Geometry: final body of the model. Coordinates: model frame, mm. Coordinates: 2 decimals unless noted, no trailing zeros. Loops run counter-clockwise (first coordinate to the right, second up) from the corner with the lowest first, then second, coordinate; pieces in that order, holes last. Notation, with made-up numbers: (76.5, 28) - (102.5, 28) arc R27 ccw to (102.5, 46) - close; hole circle Ø1 at (-28, 86.5). An arc over 180 degrees is marked (long way). Answer in a Markdown table with one row per item.
from build123d import *

# Parameters (mm, degrees)
SKETCH_1_W      = 3
SKETCH_1_H      = 30
EXTRUDE_1_DEPTH = 0.6


with BuildPart() as part:
    # Эскиз1 → Бобышка-Вытянуть1 (new body)
    with BuildSketch(Plane(origin=(0, 0, 0), x_dir=(1, 0, 0), z_dir=(0, 1, 0))):
        Polygon((0, 78), (0, 0), (98, 0), (98, 78), (50.5, 78), (50.5, 48), (47.5, 48), (47.5, 78), align=None)
        with Locations((49, 93)):
            Rectangle(SKETCH_1_W, SKETCH_1_H)
        with Locations((49, 63)):
            Rectangle(SKETCH_1_W, SKETCH_1_H)
    extrude(amount=EXTRUDE_1_DEPTH)


solid = part.part
(1) Cut plane B-B on x = 17. Output: boundary loops of the cut face in (y, z), then the cut area to 3 significant figures.
Verdict:
| item | result |
|---|---|
| outline | (0, -78) - (0.6, -78) - (0.6, 0) - (0, 0) - close |
| area | 46.8 mm² |
(2) Cut plane A-A on y = 0.5. Output: boundary loops of the cut face in (x, z).
Verdict:
| item | result |
|---|---|
| outline | (0, -78) - (47.5, -78) - (47.5, -108) - (50.5, -108) - (50.5, -78) - (98, -78) - (98, 0) - (0, 0) - close |
(3) Ray query, probe 1 along Z at (x, y) = (55.5, 0.35); probe 2 along X at (y, z) = (0.5, -87.5). Return the intervals inside material, ascending.
Verdict:
| item | result |
|---|---|
| probe 1 | z = -78 to 0 |
| probe 2 | x = 47.5 to 50.5 |
